Can you work these out from the model? Positions are in its coordinate system, mm. Give positions to 0.01 mm unless a question says otherwise; leave off trailing zeros. Loops run counter-clockwise (first coordinate to the right, second up) from the corner with the lowest first, then second, coordinate; pieces in that order, holes last. Notation, with made-up numbers: (82.5, 64.25) - (116.5, 64.25) arc R25 cw to (116.5, 101.25) - close; hole circle Ø11 at (-6, 49.25). An arc over 180 degrees is marked (long way). Answer as a JSON object with one key per item and string values. Group by question number.
Item 1: Will this pin go through, and if not, where does the flat tip stop? pin 1 (1.5 mm diameter, centred on x = 8.5, y = 3.5, fed in from +Z).
Item 2: Suppose I cut it at D-D on x = 43.5. Write out the boundary of the cut face in (y, z).
Item 3: Please list where these lines run through material, in increasing order: L1, parallel to Y at x = 44.45, z = 1.5; L2, parallel to X at y = 3.5, z = -1.5; L3, parallel to Y at x = 45.5, z = -3.
Item 4: Suppose I cut it at A-A on z = -1.5. Count the separate pieces of the cut face and the enclosed holes in it, and give its area (3 significant figures).
Item 5: Thinking about a two-plate mould opening in Z: for faces 1 (the cylindrical face through (52.728, 3.131, 1.229)), 2 (the cylindrical face through (25, 3, 0)), 3 (the flat face through (26, 3, -6.35)), 4 (the flat face through (25, 0, -2)), which applies, pulls with the +Z half, pulls with the -Z half, needs draft (parallel to the pull), parting line crosses it, or undercut?
from build123d import *

# Parameters (mm, degrees)
SKETCH1_R               = 2.286
BOSS_EXTRUDE1_DEPTH     = 6.35
CUT_EXTRUDE1_REACH      = 59.018
CUT_EXTRUDE1_END_RADIUS = 65.352083333
SKETCH2_R               = 1.905


with BuildPart() as part:
    # Sketch1 → Boss-Extrude1 (new body)
    with BuildSketch(Plane(origin=(0, 0, 0), x_dir=(1, 0, 0), z_dir=(0, 1, 0))):
        with BuildLine():
            Line((-4.7625, 6.35), (-4.7625, 0))
            ThreePointArc((-4.7625, 0), (-2.689307148, -3.930525832), (1.725283019, -4.439009434))
            ThreePointArc((1.725283019, -4.439009434), (25.4, 0), (49.074716981, -4.439009434))
            ThreePointArc((49.074716981, -4.439009434), (53.489307148, -3.930525832), (55.5625, 0))
            Line((55.5625, 0), (55.5625, 6.35))
            Line((55.5625, 6.35), (-4.7625, 6.35))
        make_face()
        with Locations(Location((0, 0, 0), (0, 0, 270))):
            Circle(SKETCH1_R, mode=Mode.SUBTRACT)
        with Locations(Location((50.8, 0, 0), (0, 0, 270))):
            Circle(SKETCH1_R, mode=Mode.SUBTRACT)
    extrude(amount=BOSS_EXTRUDE1_DEPTH)

    # Cut-Extrude1: up to this cylinder (the profile starts outside it)
    cut_extrude1_end = Plane(origin=(25.4, 3.96875, 65.352083333), z_dir=(0, -1, 0)) * Cylinder(CUT_EXTRUDE1_END_RADIUS, 249.740166667, mode=Mode.PRIVATE)
    # Sketch2 → Cut-Extrude1 (cut, up to the surface)
    with BuildSketch(Plane(origin=(0, 0, -6.35), x_dir=(-1, 0, 0), z_dir=(0, 0, -1)), mode=Mode.PRIVATE) as cut_extrude1_sk1:
        with Locations((-6.35, 3.96875)):
            Circle(SKETCH2_R)
    cut_extrude1_tool1 = extrude(cut_extrude1_sk1.sketch, amount=-CUT_EXTRUDE1_REACH, mode=Mode.PRIVATE) - cut_extrude1_end
    add(cut_extrude1_tool1.solids().sort_by_distance((6.35, 3.96875, -6.35))[0], mode=Mode.SUBTRACT)
    # Sketch2 → Cut-Extrude1 (cut, up to the surface)
    with BuildSketch(Plane(origin=(0, 0, -6.35), x_dir=(-1, 0, 0), z_dir=(0, 0, -1)), mode=Mode.PRIVATE) as cut_extrude1_sk2:
        with Locations((-44.45, 3.96875)):
            Circle(SKETCH2_R)
    cut_extrude1_tool2 = extrude(cut_extrude1_sk2.sketch, amount=-CUT_EXTRUDE1_REACH, mode=Mode.PRIVATE) - cut_extrude1_end
    add(cut_extrude1_tool2.solids().sort_by_distance((44.45, 3.96875, -6.35))[0], mode=Mode.SUBTRACT)


solid = part.part
Worked out:
{
 "1": {"pin 1": "stops at z = 2.37"},
 "2": {"outline": "(0, -6.35) - (2.32, -6.35) - (2.32, 2.56) - (0, 2.56) - close; (5.62, -6.35) - (6.35, -6.35) - (6.35, 2.56) - (5.62, 2.56) - close"},
 "3": {"L1": "y = 0 to 2.06, 5.87 to 6.35", "L2": "x = -4.76 to -1.73, 1.73 to 4.5, 8.2 to 42.6, 46.3 to 49.07, 52.53 to 55.56", "L3": "y = 0 to 2.38, 5.56 to 6.35"},
 "4": {"separate pieces": "3", "enclosed holes": "2", "area": "316 mm2"},
 "5": {"face 1": "undercut", "face 2": "pulls with the +Z half", "face 3": "pulls with the -Z half", "face 4": "needs draft"}
}
